Geometry: final body of the model. Coordinates: model frame, mm. Face numbers are marked on the shaded views. A direction names the side the tool comes from. Give positions to 0.01 mm unless a question says otherwise; leave off trailing zeros. Write each loop counter-clockwise with the first axis right and the second up, starting at its lowest first coordinate (ties: lowest second). Pieces come first, ordered by that corner, then holes.
Q1. Pin query (flat end, axial travel): pin 1 Ø3.5 at (x, z) = (-0.5, 0.5) entering from -Y; pin 2 Ø6.5 at (x, z) = (0, 0) entering from -Y; pin 3 Ø1.5 at (y, z) = (-1.5, 3) entering from -X. Return the tip coordinate at first contact, or that it passes through.
Q2. Line query: line 1 (X direction, y = -1, z = 0); line 2 (X direction, y = -11, z = 0); line 3 (Z direction, x = -0.5, y = -8.5). Output: solid intervals per line, ascending.
Q3. Section A-A (x = 0). Return the cut outline in (y, z).
Q4. Section B-B (y = 0.5). Return the cut outline in (x, z).
Q5. Section D-D (y = -4.5). Return the cut outline in (x, z), plus the area to 3 significant figures.
Q6. Reachability of the marked faces 4, 5 and 6 from +Z, -Z, +X, -X, +Y, -Y: full face, straight path, thin tool, end or side. Return the list, or none.
Q7. Section C-C (y = -12.75). Return the cut outline in (x, z).
Q8. Mould query, pull axis X, two halves, no side actions, for the marked faces 1, 2 and 3. Classes: +X half, -X half, draft (parallel to the pull), parting line (faces both ways), or undercut.
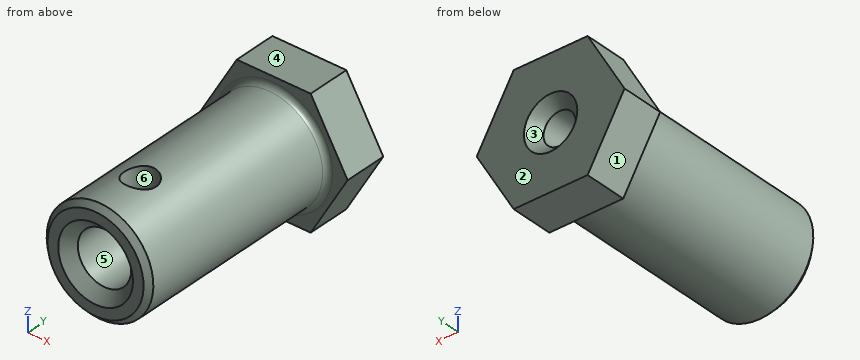
from build123d import *

# Parameters (mm, degrees)
Y_KSEKLIK_EKSTR_ZYON1_DEPTH = 4
IZIM2_R                     = 5
Y_KSEKLIK_EKSTR_ZYON2_DEPTH = 20
RADYUS3_R                   = 0.5
PAH7_SIZE                   = 0.5
IZIM4_R                     = 2.5
KES_EKSTR_ZYON3_DEPTH       = 15
IZIM3_R                     = 1.5
KES_EKSTR_ZYON4_DEPTH       = 10
IZIM8_R                     = 1.5
KES_EKSTR_ZYON5_DEPTH       = 6
PAH8_SIZE                   = 1
PAH9_SIZE                   = 1


with BuildPart() as part:
    # Çizim1 → Yükseklik-Ekstrüzyon1 (new body)
    with BuildSketch(Plane(origin=(0, 0, 0), x_dir=(1, 0, 0), z_dir=(0, 1, 0))):
        Polygon((6.92820323, 0), (3.464101615, 6), (-3.464101615, 6), (-6.92820323, 0), (-3.464101615, -6), (3.464101615, -6), align=None)
    extrude(amount=Y_KSEKLIK_EKSTR_ZYON1_DEPTH)

    # Çizim2 → Yükseklik-Ekstrüzyon2 (add)
    with BuildSketch(Plane.XZ):
        with Locations(Location((0, 0, 0), (0, 0, 270))):
            Circle(IZIM2_R)
    extrude(amount=Y_KSEKLIK_EKSTR_ZYON2_DEPTH)

    # Radyus3
    radyus3_edges = [part.edges().sort_by_distance(p)[0] for p in [
        (0, 0, 5),
    ]]
    fillet(radyus3_edges, radius=RADYUS3_R)

    # Pah7
    pah7_edges = [part.edges().sort_by_distance(p)[0] for p in [
        (0, -20, 5),
    ]]
    chamfer(pah7_edges, length=PAH7_SIZE)

    # Çizim4 → Kes-Ekstrüzyon3 (cut)
    with BuildSketch(Plane.XZ.offset(20)):
        with Locations(Location((0, 0, 0), (0, 0, 270))):
            Circle(IZIM4_R)
    extrude(amount=-KES_EKSTR_ZYON3_DEPTH, mode=Mode.SUBTRACT)

    # Çizim3 → Kes-Ekstrüzyon4 (cut)
    with BuildSketch(Plane(origin=(0, 4, 0), x_dir=(1, 0, 0), z_dir=(0, 1, 0))):
        with Locations(Location((0, 0, 0), (0, 0, 270))):
            Circle(IZIM3_R)
    extrude(amount=-KES_EKSTR_ZYON4_DEPTH, mode=Mode.SUBTRACT)

    # Çizim8 → Kes-Ekstrüzyon5 (cut)
    with BuildSketch(Plane.XY.offset(6)):
        with Locations((0, -15)):
            Circle(IZIM8_R)
    extrude(amount=-KES_EKSTR_ZYON5_DEPTH, mode=Mode.SUBTRACT)

    # Pah8
    pah8_edges = [part.edges().sort_by_distance(p)[0] for p in [
        (0, -20, 2.5),
    ]]
    chamfer(pah8_edges, length=PAH8_SIZE)

    # Pah9
    pah9_edges = [part.edges().sort_by_distance(p)[0] for p in [
        (0, 4, -1.5),
    ]]
    chamfer(pah9_edges, length=PAH9_SIZE)


solid = part.part
Computed:
1. pin 1: stops at y = -5
1. pin 2: stops at y = -19.75
1. pin 3: stops at x = -4.47
2. line 1: x = -5 to -1.5, 1.5 to 5
2. line 2: x = -5 to -2.5, 2.5 to 5
2. line 3: z = -4.97 to -2.45, 2.45 to 4.97
3. outline: (-20, -4.5) - (-19.5, -5) - (-0.5, -5) arc R0.5 cw to (0, -5.5) - (0, -6) - (4, -6) - (4, -2.5) - (3, -1.5) - (-5, -1.5) - (-5, -2.5) - (-19, -2.5) - (-20, -3.5) - close; (-20, 3.5) - (-19, 2.5) - (-16.5, 2.5) - (-16.5, 5) - (-19.5, 5) - (-20, 4.5) - close; (-13.5, 2.5) - (-5, 2.5) - (-5, 1.5) - (3, 1.5) - (4, 2.5) - (4, 6) - (0, 6) - (0, 5.5) arc R0.5 cw to (-0.5, 5) - (-13.5, 5) - close
4. outline: (-6.93, 0) - (-3.46, -6) - (3.46, -6) - (6.93, 0) - (3.46, 6) - (-3.46, 6) - close; hole circle Ø3 at (0, 0)
5. outline: circle Ø10 at (0, 0); hole circle Ø3 at (0, 0)
5. area: 71.5 mm2
6. face 4: +Z, +X, -X, +Y, -Y
6. face 5: -Y
6. face 6: +Z
7. outline: circle Ø10 at (0, 0); hole circle Ø5 at (0, 0)
8. face 1: -X half
8. face 2: draft
8. face 3: undercut
